Here's how the part is built. I have some questions about the finished solid (model axes, mm). A direction names the side the tool comes from. Give positions to 0.01 mm unless a question says otherwise; leave off trailing zeros. Write each loop counter-clockwise with the first axis right and the second up, starting at its lowest first coordinate (ties: lowest second). Pieces come first, ordered by that corner, then holes. Notation, with made-up numbers: (-9.75, 41) - (35.25, 41) arc R13 ccw to (35.25, 53) - close; hole circle Ø4 at (-39, -33.75). An arc over 180 degrees is marked (long way). Write each question's results on one line, items separated by ' | '. Start each with the question number.
Item 1: Which directions (+Z, -Z, +X, -X, +Y, -Y) give clear straight access to the entire face, cutting with the end or side of a thin tool? Please do faces 5 (the flat face through (10, 4, 0)), 6 (the cylindrical face through (-1.08, 7.01, 4.88)).
Item 2: Will this pin go through, and if not, where does the flat tip stop? P1, Ø1.8, axis at x = 0, z = 0, coming from the +Y side.
Item 3: We'd pull the mould along Z, two halves only. Please class faces 1 (the flat face through (2, 0, 0)), 2 (the flat face through (0, 4, 10)), 3 (the cylindrical face through (-0.217, 0.493, -0.976)), 4 (the flat face through (0, 4, -10)): +Z half, -Z half, draft (parallel to the pull), parting line (faces both ways), or undercut.
Item 4: Please list where these lines run through material, in increasing order: line 1 along Z through (x, y) = (0, 7.1); line 2 along Z through (x, y) = (0, 0.85).
Item 5: Suppose I cut it at A-A on y = 6.25. List the corners of the cut face in (x, z) for me.
Item 6: Suppose I cut it at C-C on x = 0. List the corners of the cut face in (y, z) for me, then the cut area to 3 significant figures.
Item 7: Suppose I cut it at D-D on x = 2.75. List the corners of the cut face in (y, z) for me.
Item 8: Suppose I cut it at B-B on z = 0. List the corners of the cut face in (x, y) for me, then the cut area to 3 significant figures.
```python
from build123d import *

# Parameters (mm, degrees)
SKETCH1_W           = 20
SKETCH1_H           = 20
BOSS_EXTRUDE1_DEPTH = 8
SKETCH2_R           = 5
CUT_EXTRUDE1_DEPTH  = 2
SKETCH3_R           = 1
CUT_EXTRUDE2_DEPTH  = 2
FILLET1_R           = 1


with BuildPart() as part:
    # Sketch1 → Boss-Extrude1 (new body)
    with BuildSketch(Plane(origin=(0, 0, 0), x_dir=(1, 0, 0), z_dir=(0, 1, 0))):
        Rectangle(SKETCH1_W, SKETCH1_H)
    extrude(amount=BOSS_EXTRUDE1_DEPTH)

    # Sketch2 → Cut-Extrude1 (cut)
    with BuildSketch(Plane(origin=(0, 8, 0), x_dir=(1, 0, 0), z_dir=(0, 1, 0))):
        Circle(SKETCH2_R)
    extrude(amount=-CUT_EXTRUDE1_DEPTH, mode=Mode.SUBTRACT)

    # Sketch3 → Cut-Extrude2 (cut)
    with BuildSketch(Plane.XZ):
        Circle(SKETCH3_R)
    extrude(amount=-CUT_EXTRUDE2_DEPTH, mode=Mode.SUBTRACT)

    # Fillet1
    fillet1_edges = [part.edges().sort_by_distance(p)[0] for p in [
        (-1, 2, 0),
    ]]
    fillet(fillet1_edges, radius=FILLET1_R)


solid = part.part
```
Checked values:
1) face 5: +Z, -Z, +X, +Y, -Y | face 6: +Y
2) P1: stops at y = 6
3) face 1: draft | face 2: +Z half | face 3: undercut | face 4: -Z half
4) line 1: z = -10 to -5, 5 to 10 | line 2: z = -10 to -1, 1 to 10
5) outline: (-10, -10) - (10, -10) - (10, 10) - (-10, 10) - close; hole circle Ø10 at (0, 0)
6) outline: (0, -10) - (8, -10) - (8, -5) - (6, -5) - (6, 5) - (8, 5) - (8, 10) - (0, 10) - (0, 1) - (1, 1) arc R1 cw to (1, -1) - (0, -1) - close | area: 136 mm^2
7) outline: (0, -10) - (8, -10) - (8, -4.18) - (6, -4.18) - (6, 4.18) - (8, 4.18) - (8, 10) - (0, 10) - close
8) outline: (-10, 0) - (-1, 0) - (-1, 1) arc R1 cw to (1, 1) - (1, 0) - (10, 0) - (10, 8) - (5, 8) - (5, 6) - (-5, 6) - (-5, 8) - (-10, 8) - close | area: 136 mm^2
